Drawing for the job (mm, zero at the part's lowest x, y, z). A direction names the side the tool comes from. Give positions to 0.01 mm unless a question says otherwise; leave off trailing zeros. One line per item, written item: value. Start each with the question number.
(1) Saw through at A-A on z = 14.5. Count the separate pieces of the cut face and the enclosed holes in it.
(2) Probe line 1 (Y direction, x = 53.5, z = 6.5); line 2 (Z direction, x = 21, y = 42) (1 decimal); line 3 (X direction, y = 10.5, z = 11.5). List the from-to ranges inside material, lowest first.
(3) Two-plate mould, pull along Y, no slides. Class the marked faces 1, 2, 3 and 4: +Y half, -Y half, draft (parallel to the pull), parting line (faces both ways), or undercut.
(4) Which spindle directions (+Z, -Z, +X, -X, +Y, -Y) get a long thin tool onto all of the face, cutting with end or side? Do the marked faces 5 and 6. Say none if no direction does.
(5) Pin check, flat tips, straight feed: pin 1 (2 mm diameter, centred on y = 17.5, z = 4.5, fed in from +X); pin 2 (4 mm diameter, centred on x = 45, z = 6.5, fed in from -Y); pin 3 (2.5 mm diameter, centred on x = 47.5, z = 2, fed in from -Y) (3 decimals); pin 4 (1.6 mm diameter, centred on y = 28.5, z = 8, fed in from +X). Stop position of each tip, or through.
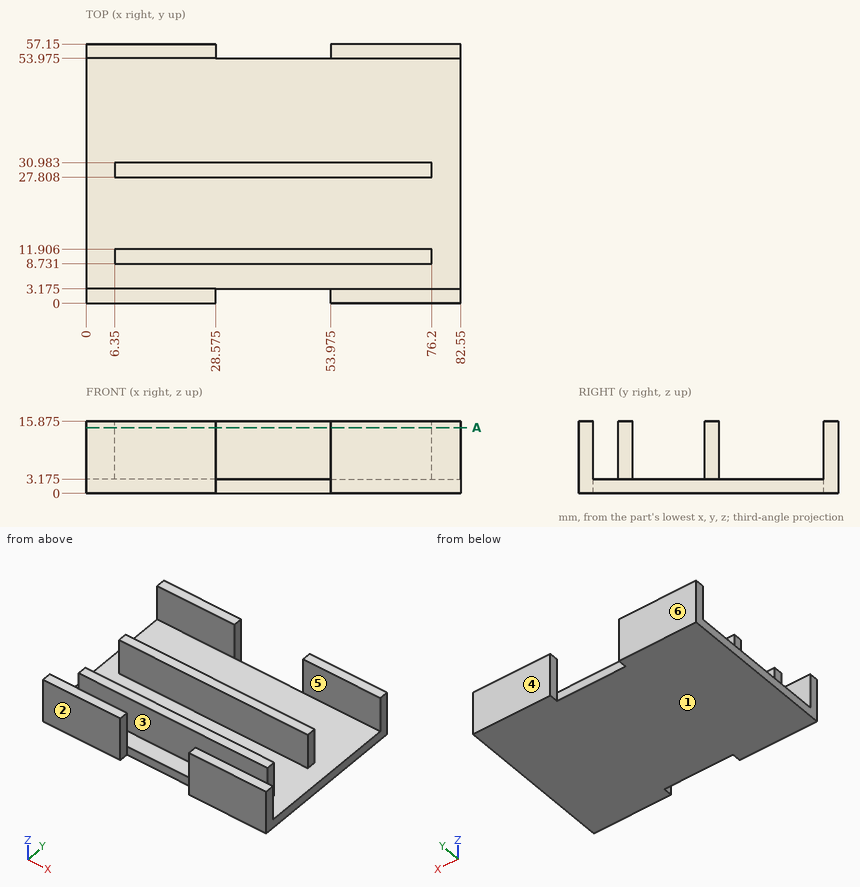
Results below:
1. separate pieces: 6
1. enclosed holes: 0
2. line 1: y = 8.73 to 11.91, 27.81 to 30.98
2. line 2: z = 0 to 3.2
2. line 3: x = 6.35 to 76.2
3. face 1: draft
3. face 2: -Y half
3. face 3: undercut
3. face 4: +Y half
4. face 5: +Z, +X, -X
4. face 6: +Z, -Z, +X, -X, +Y
5. pin 1: passes through
5. pin 2: stops at y = 8.73
5. pin 3: stops at y = 3.175
5. pin 4: stops at x = 76.2
